```python
from build123d import *

# Parameters (mm, degrees)
SKETCH1_W           = 55.5
SKETCH1_H           = 69
BOSS_EXTRUDE1_DEPTH = 9.15
FILLET1_R           = 9.15


with BuildPart() as part:
    # Sketch1 → Boss-Extrude1 (new, symmetric)
    with BuildSketch(Plane(origin=(0, 0, 0), x_dir=(1, 0, 0), z_dir=(0, 1, 0))):
        Rectangle(SKETCH1_W, SKETCH1_H)
    extrude(amount=BOSS_EXTRUDE1_DEPTH, both=True)

    # Fillet1
    fillet1_edges = [part.edges().sort_by_distance(p)[0] for p in [
        (27.75, -9.15, 0),
        (27.75, 9.15, 0),
        (-27.75, -9.15, 0),
        (-27.75, 9.15, 0),
    ]]
    fillet(fillet1_edges, radius=FILLET1_R - 0.0001)  # a hair under: the kernel refuses the full size


solid = part.part
```
Geometry check sheet. Reference: the model listing, model coordinates, mm. Coordinates: 2 decimals unless noted, no trailing zeros. Write each loop counter-clockwise with the first axis right and the second up, starting at its lowest first coordinate (ties: lowest second). Pieces come first, ordered by that corner, then holes. Notation, with made-up numbers: M 29,-0.5 L 61,-0.5 A14 cw 61,17.5 Z; hole C -26,55.5 d4. An arc over 180 degrees is marked long. One line per item, written item: value. Start each with the question number.
(1) Sectioned sample at C-C, the plane x = 22. Enter the section's corners in (y, z).
(2) Scan lines: line 1 along X through (y, z) = (-0.5, 16.5); line 2 along X through (y, z) = (-7.75, -10); line 3 along Y through (x, z) = (21, -23.5). Record each from-to range of solid material in increasing order. Write a range as [from, to].
(3) Sectioned sample at B-B, the plane y = -6.5. Enter the section's corners in (x, z), and give its area (3 significant figures).
(4) Depth check by flat-ended pin: pin 1 (1.5 mm diameter, centred on y = 6, z = -25.5, fed in from +X). Enter the tip coordinate at first touch or a pass-through.
Filled sheet:
1. outline: M -8.49,-34.5 L 8.49,-34.5 L 8.49,34.5 L -8.49,34.5 Z
2. line 1: [-27.74, 27.74]
2. line 2: [-23.46, 23.46]
2. line 3: [-8.83, 8.83]
3. outline: M -25.04,-34.5 L 25.04,-34.5 L 25.04,34.5 L -25.04,34.5 Z
3. area: 3,460 mm²
4. pin 1: x = 26.09
